Here's how the part is built. I have some questions about the finished solid (model axes, mm). A direction names the side the tool comes from. Coordinates: 2 decimals unless noted, no trailing zeros. Loops run counter-clockwise (first coordinate to the right, second up) from the corner with the lowest first, then second, coordinate; pieces in that order, holes last. Notation, with made-up numbers: (-30, -3.5) -> (0, -3.5) arc R21 cw to (0, 2.5) -> close; hole circle Ø6 at (78.25, -5.75). An arc over 180 degrees is marked (long way). Use CSV: the item, a comma, the result in double quotes. Start each with the question number.
from build123d import *

# Parameters (mm, degrees)
SKETCH_1_R      = 1.5
SKETCH_1_R_2    = 1
EXTRUDE_1_DEPTH = 2


with BuildPart() as part:
    # 草图1 → 凸台-拉伸1 (new body)
    with BuildSketch(Plane.XY):
        with BuildLine():
            Line((41.276428571, -8.854285714), (-42.723571429, -8.854285714))
            Line((-42.723571429, -8.854285714), (-42.723571429, -21.854285714))
            Line((-42.723571429, -21.854285714), (-54.723571429, -21.854285714))
            Line((-54.723571429, -21.854285714), (-54.723571429, 22.145714286))
            Line((-54.723571429, 22.145714286), (-42.723571429, 22.145714286))
            Line((-42.723571429, 22.145714286), (-42.723571429, 9.145714286))
            Line((-42.723571429, 9.145714286), (41.276428571, 9.145714286))
            ThreePointArc((41.276428571, 9.145714286), (50.276428571, 0.145714286), (41.276428571, -8.854285714))
        make_face()
        with Locations((1.276428571, 0.145714286)):
            Circle(SKETCH_1_R, mode=Mode.SUBTRACT)
        with Locations((-48.723571429, 16.645714286)):
            Circle(SKETCH_1_R, mode=Mode.SUBTRACT)
        with Locations((-48.723571429, -16.354285714)):
            Circle(SKETCH_1_R, mode=Mode.SUBTRACT)
        with Locations((41.276428571, 6.145714286)):
            Circle(SKETCH_1_R_2, mode=Mode.SUBTRACT)
        with Locations((47.276428571, 0.145714286)):
            Circle(SKETCH_1_R_2, mode=Mode.SUBTRACT)
        with Locations((41.276428571, -5.854285714)):
            Circle(SKETCH_1_R_2, mode=Mode.SUBTRACT)
        with Locations((35.276428571, 0.145714286)):
            Circle(SKETCH_1_R_2, mode=Mode.SUBTRACT)
    extrude(amount=EXTRUDE_1_DEPTH)


solid = part.part
1) For P1, Ø2.5, axis at x = 35.28, y = 0.15, coming from the -Z side; P2, Ø1.6, axis at x = 41.28, y = -5.85, coming from the -Z side; P3, Ø0.6, axis at x = 3, z = 1, coming from the -Y side, each with a flat end and sliding along its axis, tell me the tip position at first contact or that it passes through.
2) I want a section at B-B, the plane z = 0.65. Please give me the cut outline in (x, y).
3) I want a section at A-A, the plane x = -24.5. Please give me the cut outline in (y, z).
4) Which directions (+Z, -Z, +X, -X, +Y, -Y) give clear straight access to the entire face, cutting with the end or side of a thin tool? Please do faces 1 (the face through (42.23, 6.45, 0.99)), 2 (the face through (-42.724, -15, 1)), 3 (the face through (-42.724, 16, 1)).
5) Thinking about a two-plate mould opening in X: for faces 4 (the face through (-54.724, 0, 1)), 5 (the face through (48.23, 0.45, 0.99)), 6 (the face through (-49, 22.146, 1)), which applies, pulls with the +X half, pulls with the -X half, needs draft (parallel to the pull), parting line crosses it, or undercut?
6) I want a section at C-C, the plane y = -11.5. Please give me the cut outline in (x, z), plus the area to 3 significant figures.
7) Please list where these lines run through material, in increasing order: L1, parallel to Y at x = 42, z = 0.4; L2, parallel to Y at x = -5, z = 1.2; L3, parallel to X at y = 13, z = 0.7. Write a range as [from, to].
Return value:
1,P1,"stops at z = 0"
1,P2,"passes through"
1,P3,"stops at y = -8.85"
2,outline,"(-54.72, -21.85) -> (-42.72, -21.85) -> (-42.72, -8.85) -> (41.28, -8.85) arc R9 ccw to (41.28, 9.15) -> (-42.72, 9.15) -> (-42.72, 22.15) -> (-54.72, 22.15) -> close; hole circle Ø3 at (-48.72, -16.35); hole circle Ø3 at (-48.72, 16.65); hole circle Ø3 at (1.28, 0.15); hole circle Ø2 at (35.28, 0.15); hole circle Ø2 at (41.28, -5.85); hole circle Ø2 at (41.28, 6.15); hole circle Ø2 at (47.28, 0.15)"
3,outline,"(-8.85, 0) -> (9.15, 0) -> (9.15, 2) -> (-8.85, 2) -> close"
4,face 1,"+Z, -Z"
4,face 2,"+Z, -Z, +X, -Y"
4,face 3,"+Z, -Z, +X, +Y"
5,face 4,"pulls with the -X half"
5,face 5,"undercut"
5,face 6,"needs draft"
6,outline,"(-54.72, 0) -> (-42.72, 0) -> (-42.72, 2) -> (-54.72, 2) -> close"
6,area,"24.0 mm²"
7,L1,"y = [-8.83, -6.54], [-5.16, 5.46], [6.84, 9.12]"
7,L2,"y = [-8.85, 9.15]"
7,L3,"x = [-54.72, -42.72]"
